Geometry check sheet. Reference: the model listing, model coordinates, mm. Face numbers are marked on the shaded views. Give positions to 0.01 mm unless a question says otherwise; leave off trailing zeros. Write each loop counter-clockwise with the first axis right and the second up, starting at its lowest first coordinate (ties: lowest second). Pieces come first, ordered by that corner, then holes. Notation, with made-up numbers: (-23, 65) - (30, 65) arc R30 ccw to (30, 101) - close; hole circle Ø6 at (15.5, -27). An arc over 180 degrees is marked (long way). Use a Markdown table: item, result.
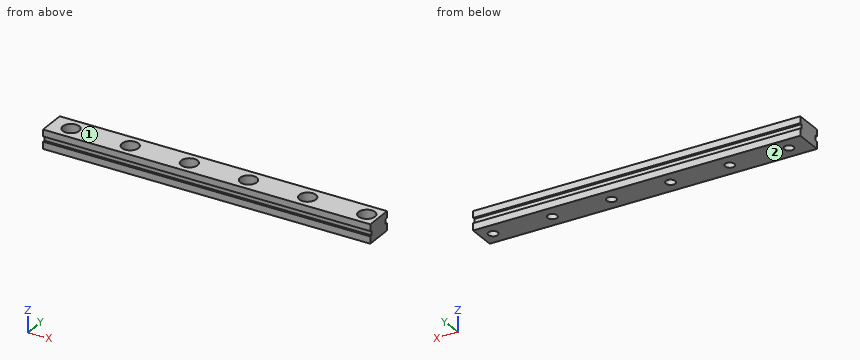
```python
from build123d import *

# Parameters (mm, degrees)
F_100_START                                  = 32.4
F_100_MM_MGN7_RAIL_7_X_4_8_MM_PROFILE_W      = 100
F_100_MM_MGN7_RAIL_7_X_4_8_MM_PROFILE_H      = 7
F_100_MM_MGN7_RAIL_7_X_4_8_MM_DEPTH          = 4.8
NOMINAL_START                                = 34.2
NOMINAL_RACEWAY_CLEARANCE_PROFILE_W          = 100.2
NOMINAL_RACEWAY_CLEARANCE_PROFILE_H          = 1.05
NOMINAL_RACEWAY_CLEARANCE_DEPTH              = 1.3
SEVEN_START                                  = 32.3
SEVEN_RAIL_MOUNTING_HOLES_15_MM_PITCH_PR_R   = 1.2
SEVEN_RAIL_MOUNTING_HOLES_15_MM_PITCH_DEPTH  = 5
M2_START                                     = 34.9
M2_RAIL_BOLT_COUNTERBORES_DIAMETER_4_2_P_R   = 2.1
M2_RAIL_BOLT_COUNTERBORES_DIAMETER_4_2_DEPTH = 2.4
SKETCH_1_W                                   = 17
SKETCH_1_H                                   = 7
CUT_EXTRUDE_1_DEPTH                          = 10


with BuildPart() as part:
    # 100 mm MGN7 rail 7 x 4.8 mm profile → 100 mm MGN7 rail 7 x 4.8 mm (new body)
    with BuildSketch(Plane.XY.offset(F_100_START)):
        with Locations((33, 19)):
            Rectangle(F_100_MM_MGN7_RAIL_7_X_4_8_MM_PROFILE_W, F_100_MM_MGN7_RAIL_7_X_4_8_MM_PROFILE_H)
    extrude(amount=F_100_MM_MGN7_RAIL_7_X_4_8_MM_DEPTH)

    # Nominal raceway clearance profile → Nominal raceway clearance (cut)
    with BuildSketch(Plane.XY.offset(NOMINAL_START)):
        with Locations((33, 15.525)):
            Rectangle(NOMINAL_RACEWAY_CLEARANCE_PROFILE_W, NOMINAL_RACEWAY_CLEARANCE_PROFILE_H)
        with Locations((33, 22.475)):
            Rectangle(NOMINAL_RACEWAY_CLEARANCE_PROFILE_W, NOMINAL_RACEWAY_CLEARANCE_PROFILE_H)
    extrude(amount=NOMINAL_RACEWAY_CLEARANCE_DEPTH, mode=Mode.SUBTRACT)

    # Seven rail mounting holes 15 mm pitch profile → Seven rail mounting holes 15 mm pitch (cut)
    with BuildSketch(Plane.XY.offset(SEVEN_START)):
        with Locations((-12, 19)):
            Circle(SEVEN_RAIL_MOUNTING_HOLES_15_MM_PITCH_PR_R)
        with Locations((3, 19)):
            Circle(SEVEN_RAIL_MOUNTING_HOLES_15_MM_PITCH_PR_R)
        with Locations((18, 19)):
            Circle(SEVEN_RAIL_MOUNTING_HOLES_15_MM_PITCH_PR_R)
        with Locations((33, 19)):
            Circle(SEVEN_RAIL_MOUNTING_HOLES_15_MM_PITCH_PR_R)
        with Locations((48, 19)):
            Circle(SEVEN_RAIL_MOUNTING_HOLES_15_MM_PITCH_PR_R)
        with Locations((63, 19)):
            Circle(SEVEN_RAIL_MOUNTING_HOLES_15_MM_PITCH_PR_R)
        with Locations((78, 19)):
            Circle(SEVEN_RAIL_MOUNTING_HOLES_15_MM_PITCH_PR_R)
    extrude(amount=SEVEN_RAIL_MOUNTING_HOLES_15_MM_PITCH_DEPTH, mode=Mode.SUBTRACT)

    # M2 rail bolt counterbores diameter 4.2 profile → M2 rail bolt counterbores diameter 4.2 (cut)
    with BuildSketch(Plane.XY.offset(M2_START)):
        with Locations((-12, 19)):
            Circle(M2_RAIL_BOLT_COUNTERBORES_DIAMETER_4_2_P_R)
        with Locations((3, 19)):
            Circle(M2_RAIL_BOLT_COUNTERBORES_DIAMETER_4_2_P_R)
        with Locations((18, 19)):
            Circle(M2_RAIL_BOLT_COUNTERBORES_DIAMETER_4_2_P_R)
        with Locations((33, 19)):
            Circle(M2_RAIL_BOLT_COUNTERBORES_DIAMETER_4_2_P_R)
        with Locations((48, 19)):
            Circle(M2_RAIL_BOLT_COUNTERBORES_DIAMETER_4_2_P_R)
        with Locations((63, 19)):
            Circle(M2_RAIL_BOLT_COUNTERBORES_DIAMETER_4_2_P_R)
        with Locations((78, 19)):
            Circle(M2_RAIL_BOLT_COUNTERBORES_DIAMETER_4_2_P_R)
    extrude(amount=M2_RAIL_BOLT_COUNTERBORES_DIAMETER_4_2_DEPTH, mode=Mode.SUBTRACT)

    # 草图1 → 切除-拉伸1 (cut)
    with BuildSketch(Plane.XY.offset(37.2)):
        with Locations((74.5, 19)):
            Rectangle(SKETCH_1_W, SKETCH_1_H)
    extrude(amount=-CUT_EXTRUDE_1_DEPTH, mode=Mode.SUBTRACT)


solid = part.part
```
1) Section check C-C on x = 21. Record the boundary of the cut face in (y, z).
Working result:
| item | result |
|---|---|
| outline | (15.5, 32.4) - (22.5, 32.4) - (22.5, 34.2) - (21.95, 34.2) - (21.95, 35.5) - (22.5, 35.5) - (22.5, 37.2) - (15.5, 37.2) - (15.5, 35.5) - (16.05, 35.5) - (16.05, 34.2) - (15.5, 34.2) - close |
2) Material ranges on L1, parallel to Z at x = 39, y = 22; L2, parallel to Y at x = 48, z = 36.5; L3, parallel to Y at x = 33, z = 33.65, recorded low to high. Write a range as from..to.
Working result:
| item | result |
|---|---|
| L1 | z = 32.4..34.2, 35.5..37.2 |
| L2 | y = 15.5..16.9, 21.1..22.5 |
| L3 | y = 15.5..17.8, 20.2..22.5 |
3) Section check B-B on x = -12. Record the boundary of the cut face in (y, z).
Working result:
| item | result |
|---|---|
| outline | (15.5, 32.4) - (17.8, 32.4) - (17.8, 34.9) - (16.9, 34.9) - (16.9, 37.2) - (15.5, 37.2) - (15.5, 35.5) - (16.05, 35.5) - (16.05, 34.2) - (15.5, 34.2) - close; (20.2, 32.4) - (22.5, 32.4) - (22.5, 34.2) - (21.95, 34.2) - (21.95, 35.5) - (22.5, 35.5) - (22.5, 37.2) - (21.1, 37.2) - (21.1, 34.9) - (20.2, 34.9) - close |
4) Depth check by flat-ended pin: P1, Ø1.4, axis at x = 63, y = 19, coming from the -Z side; P2, Ø1.3, axis at x = 32.5, y = 18.5, coming from the +Z side. Enter the tip coordinate at first touch or a pass-through.
Working result:
| item | result |
|---|---|
| P1 | passes through |
| P2 | stops at z = 34.9 |
5) Mould release check, pull along Z, two halves, no side actions. Record for the marked faces 1 and 2: pulls with the +Z half, pulls with the -Z half, needs draft (parallel to the pull), parting line crosses it, or undercut.
Working result:
| item | result |
|---|---|
| face 1 | pulls with the +Z half |
| face 2 | pulls with the -Z half |
6) Section check D-D on z = 33.25. Record the boundary of the cut face in (x, y).
Working result:
| item | result |
|---|---|
| outline | (-17, 15.5) - (66, 15.5) - (66, 22.5) - (-17, 22.5) - close; hole circle Ø2.4 at (-12, 19); hole circle Ø2.4 at (3, 19); hole circle Ø2.4 at (18, 19); hole circle Ø2.4 at (33, 19); hole circle Ø2.4 at (48, 19); hole circle Ø2.4 at (63, 19) |
7) Section check A-A on z = 36.2. Record the boundary of the cut face in (x, y), then the cut area to 3 significant figures.
Working result:
| item | result |
|---|---|
| outline | (-17, 15.5) - (66, 15.5) - (66, 22.5) - (-17, 22.5) - close; hole circle Ø4.2 at (-12, 19); hole circle Ø4.2 at (3, 19); hole circle Ø4.2 at (18, 19); hole circle Ø4.2 at (33, 19); hole circle Ø4.2 at (48, 19); hole circle Ø4.2 at (63, 19) |
| area | 498 mm² |
